Work out the finished part from the listing and answer in its coordinate system (mm). A direction names the side the tool comes from. Give positions to 0.01 mm unless a question says otherwise; leave off trailing zeros. Return JSON: item names as keys, results as strings. Group by question number.
from build123d import *

# Parameters (mm, degrees)
SKETCH1_R                   = 63.5
EXTRUDE1_DEPTH              = 6.35
SKETCH2_R                   = 58.7375
SKETCH2_R_2                 = 52.3875
EXTRUDE2_DEPTH              = 12.7
SKETCH3_W                   = 1.5875
SKETCH3_H                   = 2.38125
CHAMFER1_SIZE               = 0.5
EXTRUDE3_DEPTH              = 6.35
SKETCH4_R                   = 3.799999998
CUT_EXTRUDE1_DEPTH          = 12.7
F_6_CLEARANCE_HOLE1_D       = 3.7973
F_6_CLEARANCE_HOLE1_DEPTH   = 330.2
F_6_CLEARANCE_HOLE1_TIP     = 1.140824014
FILLET1_R                   = 6.35
M14_5_14_5_DIAMETER_HOLE1_D = 14.5
TAP_DRILL_FOR_6_TAP1_D      = 2.7051
TAP_DRILL_FOR_6_TAP1_DEPTH  = 3.302
TAP_DRILL_FOR_6_TAP1_TIP    = 0.81269403


with BuildPart() as part:
    # Sketch1 → Extrude1 (new body)
    with BuildSketch(Plane(origin=(0, 0, 0), x_dir=(1, 0, 0), z_dir=(0, 1, 0))):
        Circle(SKETCH1_R)
    extrude(amount=EXTRUDE1_DEPTH)

    # Sketch2 → Extrude2 (add)
    with BuildSketch(Plane(origin=(0, 6.35, 0), x_dir=(-1, 0, 0), z_dir=(0, 1, 0))):
        Circle(SKETCH2_R)
        Circle(SKETCH2_R_2, mode=Mode.SUBTRACT)
    extrude(amount=EXTRUDE2_DEPTH)

    # Sketch3 → Cut-Revolve1 (revolve, cut)
    with BuildSketch(Plane(origin=(0, 0, 0), x_dir=(0, 0, -1), z_dir=(1, 0, 0))):
        with Locations((-57.94375, 15.656558664)):
            Rectangle(SKETCH3_W, SKETCH3_H)
        with Locations((-57.94375, 10.842416167)):
            Rectangle(SKETCH3_W, SKETCH3_H)
    revolve(axis=Axis((0, 0, 0), (0, 1, 0)), mode=Mode.SUBTRACT)

    # Chamfer1
    chamfer1_edges = [part.edges().sort_by_distance(p)[0] for p in [
        (58.7375, 16.847183664, 0),
        (58.7375, 14.465933664, 0),
        (58.7375, 12.033041167, 0),
        (58.7375, 9.651791167, 0),
        (58.7375, 19.05, 0),
        (52.3875, 19.05, 0),
    ]]
    chamfer(chamfer1_edges, length=CHAMFER1_SIZE)

    # Sketch5 → Extrude3 (add)
    with BuildSketch(Plane.XZ):
        with BuildLine():
            Line((-69.85, 9.525), (69.85, 9.525))
            ThreePointArc((69.85, 9.525), (74.340128061, 7.665128061), (76.2, 3.175))
            Line((76.2, 3.175), (76.2, -3.175))
            ThreePointArc((76.2, -3.175), (74.340128061, -7.665128061), (69.85, -9.525))
            Line((69.85, -9.525), (-69.85, -9.525))
            ThreePointArc((-69.85, -9.525), (-74.340128061, -7.665128061), (-76.2, -3.175))
            Line((-76.2, -3.175), (-76.2, 3.175))
            ThreePointArc((-76.2, 3.175), (-74.340128061, 7.665128061), (-69.85, 9.525))
        make_face()
    extrude(amount=-EXTRUDE3_DEPTH)

    # Sketch4 → Cut-Extrude1 (cut)
    with BuildSketch(Plane.XZ):
        with Locations((-5.783711742, -36.038849572)):
            Circle(SKETCH4_R)
        with Locations((-0.38259163, -45.577892791)):
            Circle(SKETCH4_R)
        with Locations((5.17790207, -36.130863955)):
            Circle(SKETCH4_R)
    extrude(amount=-CUT_EXTRUDE1_DEPTH, mode=Mode.SUBTRACT)

    # #6 Clearance Hole1
    with Locations(Plane(origin=(-69.85, 0, 0), x_dir=(0, 0, -1), z_dir=(0, -1, 0))):
        with Locations((0, 0), (0, 139.7)):
            Hole(F_6_CLEARANCE_HOLE1_D / 2, depth=F_6_CLEARANCE_HOLE1_DEPTH)
            with Locations((0, 0, -(F_6_CLEARANCE_HOLE1_DEPTH + F_6_CLEARANCE_HOLE1_TIP / 2))):  # 118° drill point
                Cone(0, F_6_CLEARANCE_HOLE1_D / 2, F_6_CLEARANCE_HOLE1_TIP, mode=Mode.SUBTRACT)

    # Fillet1
    fillet1_edges = [part.edges().sort_by_distance(p)[0] for p in [
        (62.781560788, 3.175, -9.525),
        (-62.781560788, 3.175, -9.525),
        (-62.781560788, 3.175, 9.525),
        (62.781560788, 3.175, 9.525),
    ]]
    fillet(fillet1_edges, radius=FILLET1_R)

    # M14.5 (14.5) Diameter Hole1 (through all)
    with Locations(Plane(origin=(0, 0, 41.020671835), x_dir=(0, 0, -1), z_dir=(0, -1, 0))):
        with Locations((0, 0)):
            Hole(M14_5_14_5_DIAMETER_HOLE1_D / 2)

    # Tap Drill for #6 Tap1
    with Locations(Plane(origin=(-34.6075, 6.35, -23.495), x_dir=(0, 0, 1), z_dir=(0, 1, 0))):
        with Locations((0, 0), (46.99, 0), (46.99, 69.215), (0, 69.215)):
            Hole(TAP_DRILL_FOR_6_TAP1_D / 2, depth=TAP_DRILL_FOR_6_TAP1_DEPTH)
            with Locations((0, 0, -(TAP_DRILL_FOR_6_TAP1_DEPTH + TAP_DRILL_FOR_6_TAP1_TIP / 2))):  # 118° drill point
                Cone(0, TAP_DRILL_FOR_6_TAP1_D / 2, TAP_DRILL_FOR_6_TAP1_TIP, mode=Mode.SUBTRACT)


solid = part.part
1. Determine the mould class of faces 1 (the flat face through (-39, 12.033, 43)), 2 (the flat face through (-1, 6.35, -1)), 3 (the cylindrical face through (46.612, 17.94, -35.741)), 4 (the cylindrical face through (7.221, 3.131, -32.927)) for opening direction Z: released by +Z, released by -Z, zero draft, split by the parting line, or undercut.
2. Each of these flat-tipped pins is pushed along its axis until it touches: pin 1 (3 mm diameter, centred on x = -34.61, z = 23.5, fed in from -Y); pin 2 (4 mm diameter, centred on x = -37.5, y = 10, fed in from +Z); pin 3 (8 mm diameter, centred on y = 14, z = 43.5, fed in from +X); pin 4 (0.9 mm diameter, centred on x = 69, y = 4.5, fed in from +Z) (3 decimals). Where does it stop, or does it pass through?
3. Consider probe 1 along Z at (x, y) = (-69.85, 3) (3 decimals); probe 2 along Z at (x, y) = (0.5, 10); probe 3 along X at (y, z) = (17, -33). Determine where each line is inside the solid, lowest interval first. Write a range as from..to.
4. The part is cut by section A-A (z = 0). State how many separate pieces and enclosed holes the cut face has, and give its area (3 significant figures).
5. A tool of negligible diameter and unlimited length cuts with its end or side. For faces 5 (the flat face through (-39, 14.466, 43)), 6 (the cylindrical face through (64.029, 3.131, 10.938)), 7 (the cylindrical face through (46.612, 7.731, -35.741)), from which of +Z, -Z, +X, -X, +Y, -Y can it reach the whole face along a straight path? Write none if from no direction.
Answers:
{
 "1": {"face 1": "zero draft", "face 2": "undercut", "face 3": "split by the parting line", "face 4": "undercut"},
 "2": {"pin 1": "stops at y = 0", "pin 2": "stops at z = 46.65", "pin 3": "stops at x = 43.47", "pin 4": "stops at z = 9.525"},
 "3": {"probe 1": "z = -9.525..-1.899, 1.899..9.525", "probe 2": "z = -57.15..-52.39, 52.39..57.15", "probe 3": "x = -48.17..-40.69, 40.69..48.17"},
 "4": {"separate pieces": "3", "enclosed holes": "0", "area": "1,060 mm^2"},
 "5": {"face 5": "none", "face 6": "+Z, +X, +Y, -Y", "face 7": "+Y"}
}
